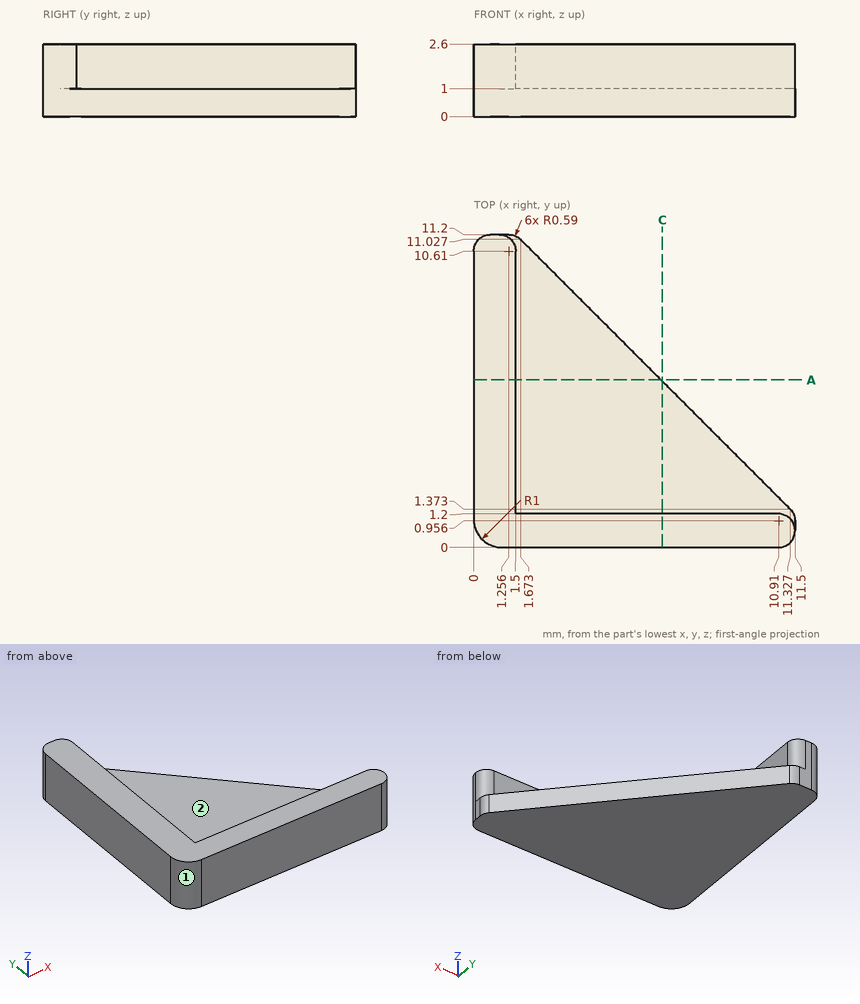
Input: dimensioned drawing with shaded views. Units: mm. Origin: part minimum x, y, z. A direction names the side the tool comes from. Coordinates: 2 decimals unless noted, no trailing zeros. Write each loop counter-clockwise with the first axis right and the second up, starting at its lowest first coordinate (ties: lowest second). Pieces come first, ordered by that corner, then holes. Notation, with made-up numbers: M 3.5,35 L 44.5,35 A25 ccw 44.5,74 Z; hole C -2.5,25 d1. An arc over 180 degrees is marked long. Answer as a JSON object with one key per item and string values. Group by question number.
(1) Contact query for flat-ended pins moving along their axis: P1, Ø0.5, axis at x = 7.5, z = 1.5, coming from the +Y side; P2, Ø0.8, axis at y = 3.5, z = 2, coming from the +X side. Output: stop coordinate, or through.
(2) Ray query, line 1 along X through (y, z) = (4, 1.9); line 2 along Y through (x, z) = (3.25, 1.05); line 3 along Z through (x, y) = (4.25, 2.5). Return the intervals inside material, ascending. Write a range as [from, to].
(3) Set-up query: the marked faces 1 and 2. Return all of +Z, -Z, +X, -X, +Y, -Y with unobstructed straight access to the full face (end or side cutting, diameter ignored); none if empty.
(4) Section C-C on x = 6.75. Output: boundary loops of the cut face in (y, z).
(5) Section A-A on y = 6. Output: boundary loops of the cut face in (x, z).
Result set:
{
 "1": {"P1": "stops at y = 1.2", "P2": "stops at x = 1.5"},
 "2": {"line 1": "x = [0, 1.5]", "line 2": "y = [0, 1.2]", "line 3": "z = [0, 1]"},
 "3": {"face 1": "+Z, -Z, -X, -Y", "face 2": "+Z, +X, +Y"},
 "4": {"outline": "M 0,0 L 5.95,0 L 5.95,1 L 1.2,1 L 1.2,2.6 L 0,2.6 Z"},
 "5": {"outline": "M 0,0 L 6.7,0 L 6.7,1 L 1.5,1 L 1.5,2.6 L 0,2.6 Z"}
}
